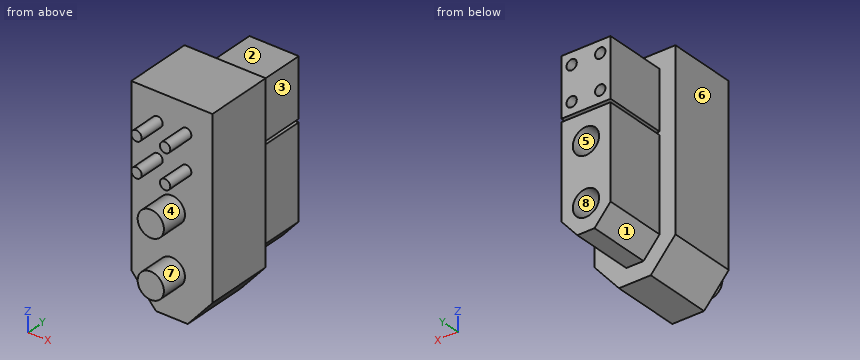
from build123d import *

# Parameters (mm, degrees)
EXTRUDE_1_DEPTH = 8.6
SKETCH_2_R      = 1.65
SKETCH_2_W      = 6.2
SKETCH_2_H      = 7.3
SKETCH_2_R_2    = 0.65
EXTRUDE_2_DEPTH = 7.9
SKETCH_3_R      = 1.65
SKETCH_3_R_2    = 0.65
EXTRUDE_3_DEPTH = 12


with BuildPart() as part:
    # 草图1 → 凸台-拉伸1 (new body)
    with BuildSketch(Plane(origin=(0, 0, 0), x_dir=(1, 0, 0), z_dir=(0, 1, 0))):
        Polygon((0, 0), (0, 22), (3.1, 25.6), (7.1, 25.6), (10.2, 22), (10.2, 0), align=None)
    extrude(amount=EXTRUDE_1_DEPTH)

    # 草图2 → 凸台-拉伸2 (add)
    with BuildSketch(Plane(origin=(0, 8.6, 0), x_dir=(1, 0, 0), z_dir=(0, 1, 0))):
        Polygon((2, 9.7), (8.2, 9.7), (8.2, 21.257555221), (6.182894773, 23.6), (4.017105227, 23.6), (2, 21.257555221), align=None)
        with Locations((5.1, 20.25)):
            Circle(SKETCH_2_R, mode=Mode.SUBTRACT)
        with Locations((5.1, 13.05)):
            Circle(SKETCH_2_R, mode=Mode.SUBTRACT)
        with Locations((5.1, 5.65)):
            Rectangle(SKETCH_2_W, SKETCH_2_H)
        with Locations((3.3, 7.8)):
            Circle(SKETCH_2_R_2, mode=Mode.SUBTRACT)
        with Locations((6.9, 7.8)):
            Circle(SKETCH_2_R_2, mode=Mode.SUBTRACT)
        with Locations((6.9, 3.5)):
            Circle(SKETCH_2_R_2, mode=Mode.SUBTRACT)
        with Locations((3.3, 3.5)):
            Circle(SKETCH_2_R_2, mode=Mode.SUBTRACT)
    extrude(amount=EXTRUDE_2_DEPTH)

    # 草图3 → 凸台-拉伸3 (add)
    with BuildSketch(Plane(origin=(0, 8.6, 0), x_dir=(1, 0, 0), z_dir=(0, 1, 0))):
        with Locations((5.1, 20.25)):
            Circle(SKETCH_3_R)
        with Locations((5.1, 13.05)):
            Circle(SKETCH_3_R)
        with Locations((3.3, 7.8)):
            Circle(SKETCH_3_R_2)
        with Locations((6.9, 7.8)):
            Circle(SKETCH_3_R_2)
        with Locations((6.9, 3.5)):
            Circle(SKETCH_3_R_2)
        with Locations((3.3, 3.5)):
            Circle(SKETCH_3_R_2)
    extrude(amount=-EXTRUDE_3_DEPTH)


solid = part.part
Can you work these out from the model? Positions are in its coordinate system, mm. Face numbers are marked on the shaded views. A direction names the side the tool comes from. Give positions to 0.01 mm unless a question says otherwise; leave off trailing zeros. Loops run counter-clockwise (first coordinate to the right, second up) from the corner with the lowest first, then second, coordinate; pieces in that order, holes last. Notation, with made-up numbers: M -31.75,-31.5 L -24.75,-31.5 A18 ccw -24.75,-18.5 Z; hole C 30.5,-11.5 d3. An arc over 180 degrees is marked long. One line per item, written item: value.
1) Imagine slicing it at B-B on y = -1.75. Write out the boundary of the cut face in (x, z), and give its area (3 significant figures).
Geometry check:
outline: C 3.3,-7.8 d1.3; C 3.3,-3.5 d1.3; C 5.1,-20.25 d3.3; C 5.1,-13.05 d3.3; C 6.9,-7.8 d1.3; C 6.9,-3.5 d1.3
area: 22.4 mm²
2) Imagine slicing it at C-C on z = -7.8. Write out the boundary of the cut face in (x, y), and give its area (3 significant figures).
Geometry check:
outline: M 0,0 L 2.65,0 L 2.65,-3.4 L 3.95,-3.4 L 3.95,0 L 6.25,0 L 6.25,-3.4 L 7.55,-3.4 L 7.55,0 L 10.2,0 L 10.2,8.6 L 8.2,8.6 L 8.2,16.5 L 7.55,16.5 L 7.55,8.6 L 6.25,8.6 L 6.25,16.5 L 3.95,16.5 L 3.95,8.6 L 2.65,8.6 L 2.65,16.5 L 2,16.5 L 2,8.6 L 0,8.6 Z
area: 125 mm²
3) Imagine slicing it at D-D on x = 5.1. Write out the boundary of the cut face in (y, z), and give its area (3 significant figures).
Geometry check:
outline: M -3.4,-21.9 L 0,-21.9 L 0,-25.6 L 8.6,-25.6 L 8.6,-23.6 L 16.5,-23.6 L 16.5,-21.9 L 8.6,-21.9 L 8.6,-18.6 L 16.5,-18.6 L 16.5,-14.7 L 8.6,-14.7 L 8.6,-11.4 L 16.5,-11.4 L 16.5,-9.7 L 8.6,-9.7 L 8.6,-9.3 L 16.5,-9.3 L 16.5,-2 L 8.6,-2 L 8.6,0 L 0,0 L 0,-11.4 L -3.4,-11.4 L -3.4,-14.7 L 0,-14.7 L 0,-18.6 L -3.4,-18.6 Z
area: 358 mm²
4) I'm going to push flat-ended pins straight in: pin 1 (1 mm diameter, centred on y = 12, z = -17.5, fed in from +X); pin 2 (1.9 mm diameter, centred on x = 5.5, y = 12, fed in from -Z); pin 3 (1.6 mm diameter, centred on x = 4.5, z = -12.5, fed in from +Y). Where does each tip first touch, or does it pass through?
Geometry check:
pin 1: stops at x = 8.2
pin 2: stops at z = -23.6
pin 3: stops at y = 8.6
5) Thinking about a two-plate mould opening in X: for the marked faces 5, 6, 7 and 8, which applies, +X half, -X half, draft (parallel to the pull), parting line (faces both ways), or undercut?
Geometry check:
face 5: undercut
face 6: -X half
face 7: parting line
face 8: undercut
6) On a 3-axis mill with a long thin cutter (end or side, diameter ignored), from which of +Z, -Z, +X, -X, +Y, -Y can I reach the whole of each face in a straight line? I mean the marked faces 1, 2, 3 and 4. Say none if no direction works.
Geometry check:
face 1: -Z, -X, +Y
face 2: +Z, +X, -X, +Y
face 3: +Z, -Z, +X, +Y
face 4: -Y
7) Please list where these lines run through material, in increasing order: line 1 (X direction, y = 13.5, z = -3.5); line 2 (Z direction, x = 5, y = 9.75); line 3 (Y direction, x = 5.75, z = -1.25).
Geometry check:
line 1: x = 2 to 2.65, 3.95 to 6.25, 7.55 to 8.2
line 2: z = -23.6 to -21.9, -18.6 to -14.7, -11.4 to -9.7, -9.3 to -2
line 3: y = 0 to 8.6
8) Imagine slicing it at A-A on y = 11. Write out the boundary of the cut face in (x, z).
Geometry check:
outline: M 2,-21.26 L 4.02,-23.6 L 6.18,-23.6 L 8.2,-21.26 L 8.2,-9.7 L 2,-9.7 Z; M 2,-9.3 L 8.2,-9.3 L 8.2,-2 L 2,-2 Z; hole C 3.3,-7.8 d1.3; hole C 3.3,-3.5 d1.3; hole C 5.1,-20.25 d3.3; hole C 5.1,-13.05 d3.3; hole C 6.9,-7.8 d1.3; hole C 6.9,-3.5 d1.3
